Design review of the part built by this model. Coordinates are the model's own, in mm. Face numbers are marked on the shaded views. A direction names the side the tool comes from. Give positions to 0.01 mm unless a question says otherwise; leave off trailing zeros. Order: outer loops, then holes, each group sorted by start corner. A loop starts at its lowest first (then second) coordinate and runs counter-clockwise, first axis right, second up. Notation, with made-up numbers: (77.5, 81) -> (134.5, 81) arc R19 ccw to (134.5, 99) -> close; hole circle Ø8 at (33, 68). An arc over 180 degrees is marked (long way). Return JSON: item names as keys, results as strings.
```python
from build123d import *

# Parameters (mm, degrees)
F1_DEPTH = 1180
F4_DEPTH = 100.001
F5_DEPTH = 100.001


with BuildPart() as f1:
    # F0 (on Front) → F1 (new body)
    with BuildSketch(Plane.XZ):
        with BuildLine():
            ThreePointArc((50, 45), (48.5355339059, 48.5355339059), (45, 50))
            Line((45, 50), (-45, 50))
            ThreePointArc((-45, 50), (-48.5355339059, 48.5355339059), (-50, 45))
            Line((-50, 45), (-50, -45))
            ThreePointArc((-50, -45), (-48.5355339059, -48.5355339059), (-45, -50))
            Line((-45, -50), (45, -50))
            ThreePointArc((45, -50), (48.5355339059, -48.5355339059), (50, -45))
            Line((50, -45), (50, 45))
        make_face()
        with BuildLine():
            ThreePointArc((-47, 45), (-46.4142135624, 46.4142135624), (-45, 47))
            Line((-45, 47), (45, 47))
            ThreePointArc((45, 47), (46.4142135624, 46.4142135624), (47, 45))
            Line((47, 45), (47, -45))
            ThreePointArc((47, -45), (46.4142135624, -46.4142135624), (45, -47))
            Line((45, -47), (-45, -47))
            ThreePointArc((-45, -47), (-46.4142135624, -46.4142135624), (-47, -45))
            Line((-47, -45), (-47, 45))
        make_face(mode=Mode.SUBTRACT)
    extrude(amount=-F1_DEPTH)

    # F3 (on offset) → F4 (cut, through all)
    with BuildSketch(Plane.XY.offset(50)):
        Polygon((-50, 100), (-50, 0), (50, 0), align=None)
    extrude(amount=-F4_DEPTH, mode=Mode.SUBTRACT)

    # F3 (on offset) → F5 (cut, through all)
    with BuildSketch(Plane.XY.offset(50)):
        Polygon((-50, 100), (-50, 0), (50, 0), align=None)
        Polygon((50, 1180), (-50, 1180), (-50, 1080), align=None)
    extrude(amount=-F5_DEPTH, mode=Mode.SUBTRACT)


solid = f1.part
```
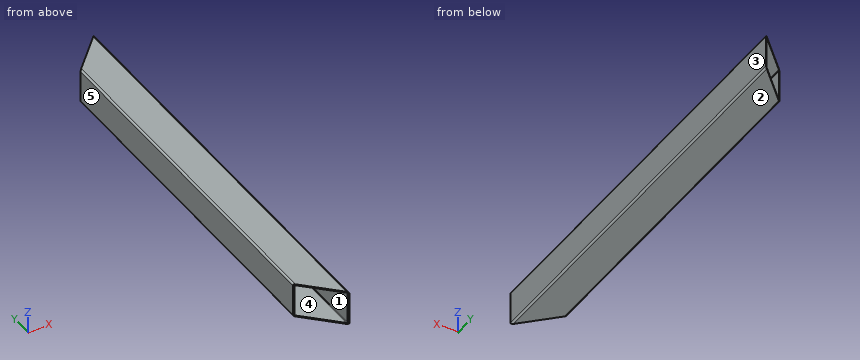
Item 1: Mouldability with a two-part tool opening along Z and no side actions: class the marked faces 1, 2 and 3 as released by +Z, released by -Z, zero draft, split by the parting line, or undercut.
Result set:
{"face 1": "undercut", "face 2": "released by -Z", "face 3": "zero draft"}
Item 2: Machinability: for the marked faces 4 and 5, which of the approach directions +Z, -Z, +X, -X, +Y, -Y give a long, thin tool a straight path to every point of the face, cutting with its end or side? Answer none if there is none.
Result set:
{"face 4": "+Y, -Y", "face 5": "+Z, -Z, -X, +Y, -Y"}
Item 3: Wall thickness on L1, parallel to X at y = 391.5, z = 36; L2, parallel to X at y = 67, z = 43.5: over which ranges is each line inside the solid? List them lowest first. Write a range as [from, to].
Result set:
{"L1": "x = [-50, -47], [47, 50]", "L2": "x = [47, 50]"}
Item 4: Add section A-A (x = -7). Give the boundary of the cut face in (y, z).
Result set:
{"outline": "(57, -50) -> (1123, -50) -> (1123, -47) -> (57, -47) -> close; (57, 47) -> (1123, 47) -> (1123, 50) -> (57, 50) -> close"}
Item 5: Add section B-B (y = 208). Give the boundary of the cut face in (x, z), plus the area to 3 significant figures.
Result set:
{"outline": "(-50, -45) arc R5 ccw to (-45, -50) -> (45, -50) arc R5 ccw to (50, -45) -> (50, 45) arc R5 ccw to (45, 50) -> (-45, 50) arc R5 ccw to (-50, 45) -> close; hole (-47, -45) arc R2 ccw to (-45, -47) -> (45, -47) arc R2 ccw to (47, -45) -> (47, 45) arc R2 ccw to (45, 47) -> (-45, 47) arc R2 ccw to (-47, 45) -> close", "area": "1,150 mm^2"}
Item 6: Add section C-C (z = -0.5). Give the boundary of the cut face in (x, y), plus the area to 3 significant figures.
Result set:
{"outline": "(-50, 100) -> (-47, 97) -> (-47, 1083) -> (-50, 1080) -> close; (47, 3) -> (50, 0) -> (50, 1180) -> (47, 1177) -> close", "area": "6,480 mm^2"}
